Geometry check sheet. Reference: the model listing, model coordinates, mm. A direction names the side the tool comes from. Round coordinates to 2 decimals unless told otherwise and drop trailing zeros. Loops run counter-clockwise (first coordinate to the right, second up) from the corner with the lowest first, then second, coordinate; pieces in that order, holes last. Notation, with made-up numbers: M 76,69.5 L 135,69.5 A21 ccw 135,91.5 Z; hole C -15,7 d9. An arc over 180 degrees is marked long. Use one line per item in the form item = value. Start each with the question number.
1. Cross-section at C-C (x = -72). Record the boundary of the cut face in (y, z).
2. Set-up check for faces 5 (the flat face through (-133, 13.391, -2)), 6 (the flat face through (-65, 0, 50)), 7 (the flat face through (-13.391, 0, 103)), 8 (the flat face through (-66, 6, -1.984)), 9 (the cylindrical face through (0.867, 23.946, 4.028)): record each of +Z, -Z, +X, -X, +Y, -Y from which the full face is reachable in a straight line by a thin tool's end or side.
3. Cross-section at A-A (z = 50.8). Record the boundary of the cut face in (x, y).
4. Draft check along X on faces 1 (the flat face through (-3.1, -0.3, 101.6)), 2 (the flat face through (-5.897, 17.304, 104.426)), 3 (the cylindrical face through (-128.045, 25.237, -2.85)), 4 (the cylindrical face through (0.6, 21.22, -2.64)). Enter one of: pulls with the +X half, pulls with the -X half, needs draft (parallel to the pull), parting line crosses it, or undercut.
5. Material ranges on line 1 (X direction, y = 13.5, z = 4.5); line 2 (Z direction, x = -113, y = 7.5); line 3 (Y direction, x = -45.5, z = 70.5), recorded low to high.
6. Cross-section at B-B (z = 35). Record the boundary of the cut face in (x, y).
7. Go/stop test with flat-tipped pins: pin 1 (0.9 mm diameter, centred on y = -0.5, z = 17.5, fed in from +X); pin 2 (4.5 mm diameter, centred on x = -126.69, y = 25.3, fed in from -Z); pin 3 (0.5 mm diameter, centred on x = -77, z = -3, fed in from +Y); pin 4 (3 mm diameter, centred on x = -24.65, z = 7.14, fed in from +Y). Record where each tip stops, or that it passes through.
```python
from build123d import *

# Parameters (mm, degrees)
F1_DEPTH  = 101.6
F2_W      = 1.70942
F2_H      = 15.875
F2_W_2    = 105.865218
F2_H_2    = 1.70942
F3_DEPTH  = 3.69316
F4_W      = 1.70942
F4_H      = 15.875
F4_W_2    = 105.865218
F4_H_2    = 1.70942
F5_DEPTH  = 3.69316
F6_W      = 105.865218
F6_H      = 1.70942
F7_DEPTH  = 9.92124
F8_W      = 15.875
F8_H      = 1.70942
F9_DEPTH  = 9.92124
F10_W     = 15.875
F10_H     = 1.70942
F11_DEPTH = 9.92124
F12_R     = 1.98374
F13_R     = 3.69316
F14_SIZE  = 7.9375
F15_R     = 1.35255
F16_DEPTH = 108.98632
F17_R     = 0.762
F18_R     = 1.35255
F19_DEPTH = 1.70942
F20_W     = 9.532924
F20_H     = 24
F20_R     = 1.35255
F21_DEPTH = 1.70942
F22_R     = 1.7272
F23_DEPTH = 1.70942


with BuildPart() as f1:
    # F0 (on Top) → F1 (new body)
    with BuildSketch(Plane.XY):
        Polygon((0, 29.265601), (0, 0), (-132.64642, 0), (-132.64642, 29.265601), (-134.35584, 29.265601), (-134.35584, -1.70942), (1.70942, -1.70942), (1.70942, 29.265601), align=None)
    extrude(amount=F1_DEPTH)

    # F2 (on face) → F3 (join)
    with BuildSketch(Plane(origin=(0, 0, 0), x_dir=(1, 0, 0), z_dir=(0, 0, -1))):
        with Locations((0.85471, -21.328101)):
            Rectangle(F2_W, F2_H)
        with Locations((-66.32321, 0.85471)):
            Rectangle(F2_W_2, F2_H_2)
        with Locations((-133.50113, -21.328101)):
            Rectangle(F2_W, F2_H)
    extrude(amount=F3_DEPTH)

    # F4 (on face) → F5 (join)
    with BuildSketch(Plane.XY.offset(101.6)):
        with Locations((-133.50113, 21.328101)):
            Rectangle(F4_W, F4_H)
        with Locations((0.85471, 21.328101)):
            Rectangle(F4_W, F4_H)
        with Locations((-66.32321, -0.85471)):
            Rectangle(F4_W_2, F4_H_2)
    extrude(amount=F5_DEPTH)

    # F6 (on face) → F7 (join)
    with BuildSketch(Plane(origin=(0, 0, 0), x_dir=(-1, 0, 0), z_dir=(0, 1, 0))):
        with Locations((66.32321, -2.83845)):
            Rectangle(F6_W, F6_H)
        with Locations((66.32321, 104.43845)):
            Rectangle(F6_W, F6_H)
    extrude(amount=F7_DEPTH)

    # F8 (on face) → F9 (join)
    with BuildSketch(Plane.YZ.offset(-132.64642)):
        with Locations((21.328101, 104.43845)):
            Rectangle(F8_W, F8_H)
        with Locations((21.328101, -2.83845)):
            Rectangle(F8_W, F8_H)
    extrude(amount=F9_DEPTH)

    # F10 (on face) → F11 (join)
    with BuildSketch(Plane(origin=(0, 0, 0), x_dir=(0, -1, 0), z_dir=(-1, 0, 0))):
        with Locations((-21.328101, -2.83845)):
            Rectangle(F10_W, F10_H)
        with Locations((-21.328101, 104.43845)):
            Rectangle(F10_W, F10_H)
    extrude(amount=F11_DEPTH)

    # F12
    f12_edges = [f1.edges().sort_by_distance(p)[0] for p in [
        (0, 21.328101, 103.58374),
        (-66.32321, 0, 103.58374),
        (-132.64642, 21.328101, 103.58374),
        (-132.64642, 21.328101, -1.98374),
        (-66.32321, 0, -1.98374),
        (0, 21.328101, -1.98374),
        (0, 0, 50.8),
        (-132.64642, 0, 50.8),
    ]]
    fillet(f12_edges, radius=F12_R)

    # F13
    f13_edges = [f1.edges().sort_by_distance(p)[0] for p in [
        (-134.35584, 21.328101, -3.69316),
        (-66.32321, -1.70942, -3.69316),
        (-134.35584, -1.70942, 50.8),
        (-66.32321, -1.70942, 105.29316),
        (-134.35584, 21.328101, 105.29316),
        (1.70942, 21.328101, -3.69316),
        (1.70942, -1.70942, 50.8),
        (1.70942, 21.328101, 105.29316),
    ]]
    fillet(f13_edges, radius=F13_R)

    # F14
    f14_edges = [f1.edges().sort_by_distance(p)[0] for p in [
        (-122.72518, 13.390601, 104.43845),
        (-119.255819, 9.92124, 104.43845),
        (-13.390601, 9.92124, 104.43845),
        (-9.92124, 13.390601, 104.43845),
        (-13.390601, 9.92124, -2.83845),
        (-9.92124, 13.390601, -2.83845),
        (-122.72518, 13.390601, -2.83845),
        (-119.255819, 9.92124, -2.83845),
    ]]
    chamfer(f14_edges, length=F14_SIZE)

    # F15 (on face) → F16 (cut, through all)
    with BuildSketch(Plane(origin=(0, 0, -3.69316), x_dir=(1, 0, 0), z_dir=(0, 0, -1))):
        with Locations((-25.296851, -5.95249)):
            Circle(F15_R)
        with Locations((-107.349569, -5.95249)):
            Circle(F15_R)
        with Locations((-126.69393, -25.296851)):
            Circle(F15_R)
        with Locations((-5.95249, -25.296851)):
            Circle(F15_R)
    extrude(amount=-F16_DEPTH, mode=Mode.SUBTRACT)

    # F17
    f17_edges = [f1.edges().sort_by_distance(p)[0] for p in [
        (-122.72518, 29.265601, -2.83845),
        (-122.72518, 29.265601, 104.43845),
        (-9.92124, 29.265601, 104.43845),
        (-9.92124, 29.265601, -2.83845),
    ]]
    fillet(f17_edges, radius=F17_R)

    # F18 (on face) → F19 (cut, through all)
    with BuildSketch(Plane.YZ.offset(1.70942)):
        with Locations((25.296851, 97.63125)):
            Circle(F18_R)
        with Locations((25.296851, 3.96875)):
            Circle(F18_R)
        with Locations((5.95249, 3.96875)):
            Circle(F18_R)
        with Locations((5.95249, 97.63125)):
            Circle(F18_R)
    extrude(amount=-F19_DEPTH, mode=Mode.SUBTRACT)

    # F20 (on face) → F21 (cut, through all)
    with BuildSketch(Plane.XZ.offset(1.70942)):
        with Locations((-9.48374, 15.175)):
            Rectangle(F20_W, F20_H)
        with Locations((-123.16268, 15.175)):
            Rectangle(F20_W, F20_H)
        with Locations((-123.16268, 86.425)):
            Rectangle(F20_W, F20_H)
        with Locations((-9.48374, 86.425)):
            Rectangle(F20_W, F20_H)
        with Locations((-24.64566, 7.14375)):
            Circle(F20_R)
        with Locations((-108.00076, 7.14375)):
            Circle(F20_R)
        with Locations((-108.00076, 94.45625)):
            Circle(F20_R)
        with Locations((-24.64566, 94.45625)):
            Circle(F20_R)
    extrude(amount=-F21_DEPTH, mode=Mode.SUBTRACT)

    # F22 (on face) → F23 (cut, through all)
    with BuildSketch(Plane(origin=(-134.35584, 0, 0), x_dir=(0, -1, 0), z_dir=(-1, 0, 0))):
        with Locations((-14.632788, 50.8)):
            Circle(F22_R)
    extrude(amount=-F23_DEPTH, mode=Mode.SUBTRACT)


solid = f1.part
```
Reported:
q1.outline = M -1.71,0 A3.69 ccw 1.98,-3.69 L 9.92,-3.69 L 9.92,-1.98 L 1.98,-1.98 A1.98 cw 0,0 L 0,101.6 A1.98 cw 1.98,103.58 L 9.92,103.58 L 9.92,105.29 L 1.98,105.29 A3.69 ccw -1.71,101.6 Z
q2.face_5 = -Z, +X, -X, -Y
q2.face_6 = +Y
q2.face_7 = +Z, +X, +Y, -Y
q2.face_8 = +X, -X, +Y
q2.face_9 = +X
q3.outline = M -134.36,1.98 A3.69 ccw -130.66,-1.71 L -1.98,-1.71 A3.69 ccw 1.71,1.98 L 1.71,29.27 L 0,29.27 L 0,1.98 A1.98 cw -1.98,0 L -130.66,0 A1.98 cw -132.65,1.98 L -132.65,12.91 L -134.36,12.91 Z; M -134.36,16.36 L -132.65,16.36 L -132.65,29.27 L -134.36,29.27 Z
q4.face_1 = needs draft
q4.face_2 = undercut
q4.face_3 = undercut
q4.face_4 = pulls with the +X half
q5.line_1 = -134.36 to -132.65, 0 to 1.71
q5.line_2 = -3.69 to -1.98, 103.58 to 105.29
q5.line_3 = -1.71 to 0
q6.outline = M -134.36,1.98 A3.69 ccw -130.66,-1.71 L -1.98,-1.71 A3.69 ccw 1.71,1.98 L 1.71,29.27 L 0,29.27 L 0,1.98 A1.98 cw -1.98,0 L -130.66,0 A1.98 cw -132.65,1.98 L -132.65,29.27 L -134.36,29.27 Z
q7.pin_1 = 1.1
q7.pin_2 = -3.69
q7.pin_3 = 9.92
q7.pin_4 = 0
